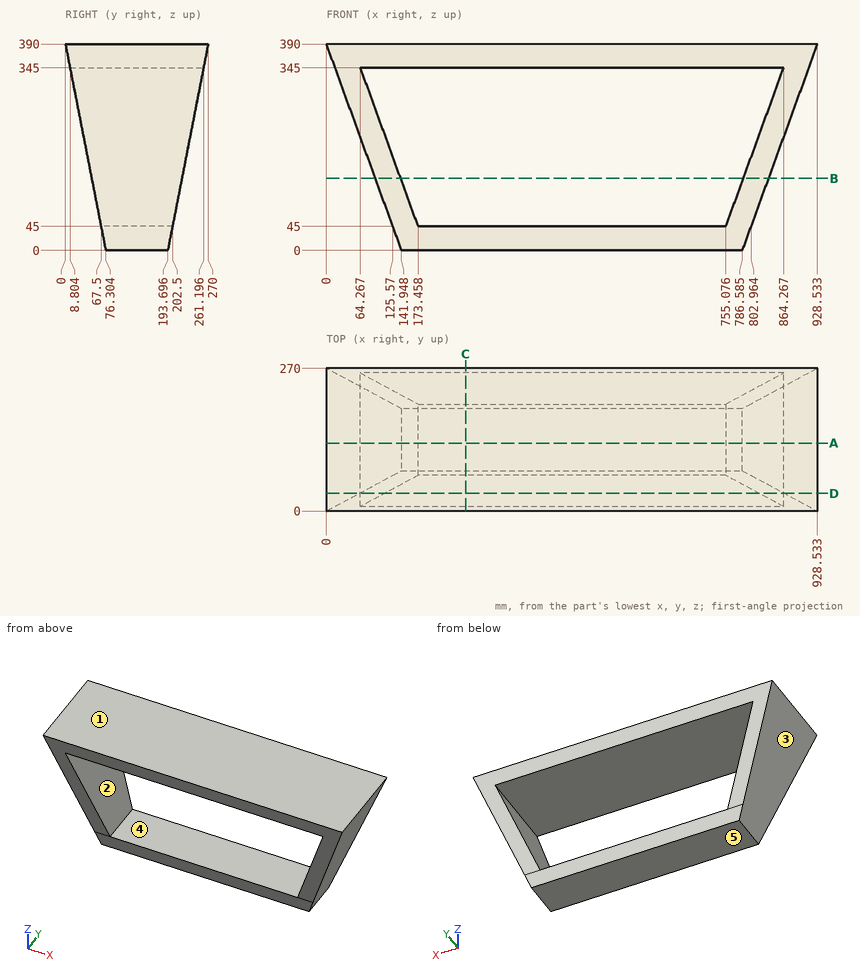
Geometry: see drawing. Coordinates: mm, zero at the bounding-box minimum. A direction names the side the tool comes from. Coordinates: 2 decimals unless noted, no trailing zeros. Write each loop counter-clockwise with the first axis right and the second up, starting at its lowest first coordinate (ties: lowest second). Pieces come first, ordered by that corner, then holes.
1) Section C-C on x = 263.5. Output: boundary loops of the cut face in (y, z) (1 decimal), and give its area (3 significant figures).
2) Section D-D on y = 33.5. Output: boundary loops of the cut face in (x, z) (1 decimal), and give its area (3 significant figures).
3) Mould query, pull axis X, two halves, no side actions, for the marked faces 3, 4 and 5. Classes: pulls with the +X half, pulls with the -X half, needs draft (parallel to the pull), parting line crosses it, or undercut.
4) Set-up query: the marked faces 1 and 2. Return all of +Z, -Z, +X, -X, +Y, -Y with unobstructed straight access to the full face (end or side cutting, diameter ignored); none if empty.
5) Section A-A on y = 128.5. Output: boundary loops of the cut face in (x, z) (1 decimal).
6) Pin query (flat end, axial travel): pin 1 Ø1.5 at (y, z) = (89.5, 171) entering from +X; pin 2 Ø6 at (x, y) = (744, 241.5) entering from -Z; pin 3 Ø5 at (y, z) = (169, 150.5) entering from +X. Return the tip coordinate at first contact, or that it passes through.
7) Material intervals for line 1 along Z through (x, y) = (550, 80.5); line 2 along X through (y, z) = (96, 50.5) (1 decimal); line 3 along X through (y, z) = (230, 281), sorted ascending.
8) Section B-B on z = 136. Output: boundary loops of the cut face in (x, y) (1 decimal), and give its area (3 significant figures).
Check result:
1. outline: (0, 390) - (8.8, 345) - (261.2, 345) - (270, 390) - close; (67.5, 45) - (76.3, 0) - (193.7, 0) - (202.5, 45) - close
1. area: 17,400 mm2
2. outline: (0, 390) - (62.3, 218.8) - (110.2, 218.8) - (64.3, 345) - (864.3, 345) - (818.3, 218.8) - (866.2, 218.8) - (928.5, 390) - close
2. area: 53,100 mm2
3. face 3: pulls with the -X half
3. face 4: undercut
3. face 5: needs draft
4. face 1: +Z, +X, -X, +Y, -Y
4. face 2: +Y, -Y
5. outline: (0, 390) - (141.9, 0) - (786.6, 0) - (928.5, 390) - close; hole (64.3, 345) - (173.5, 45) - (755.1, 45) - (864.3, 345) - close
6. pin 1: stops at x = 849.1
6. pin 2: stops at z = 345
6. pin 3: stops at x = 842.27
7. line 1: z = 0 to 45, 345 to 390
7. line 2: x = 123.6 to 171.5, 757.1 to 805
7. line 3: x = 39.67 to 87.56, 840.97 to 888.86
8. outline: (92.4, 49.7) - (140.3, 49.7) - (140.3, 220.3) - (92.4, 220.3) - close; (788.2, 49.7) - (836.1, 49.7) - (836.1, 220.3) - (788.2, 220.3) - close
8. area: 16,300 mm2
